Read the model definition and answer for the solid it produces. Units are mm, in the model's axes. A direction names the side the tool comes from. Coordinates: 2 decimals unless noted, no trailing zeros. Write each loop counter-clockwise with the first axis right and the second up, starting at its lowest first coordinate (ties: lowest second). Pieces come first, ordered by that corner, then holes.
Item 1: Each of these flat-tipped pins is pushed along its axis until it touches: P1, Ø1.9, axis at x = 0.5, y = -1, coming from the +Z side; P2, Ø1, axis at y = 1, z = -4, coming from the +X side. Where does it stop, or does it pass through?
Item 2: Section C-C (z = 2.25) is taken. Give the vertices of the cut face in (x, y), then the cut area to 3 significant figures.
Item 3: Section D-D (z = -10.75) is taken. Give the vertices of the cut face in (x, y).
Item 4: Determine the mould class of faces 1 (the face through (6.221, 0.028, 8.113)), 2 (the face through (-4.3, 2.032, 9.5)), 3 (the face through (0, 0, -12.7)), 4 (the face through (5, 0, 12.7)) for opening direction Z: released by +Z, released by -Z, zero draft, split by the parting line, or undercut.
Item 5: Straight lines are drawn through the part: probe 1 along X at (y, z) = (-0.2, 7.75); probe 2 along X at (y, z) = (0.4, 6.5); probe 3 along Z at (x, y) = (9, 1.3). For each, find the intervals that lie inside material, in ascending order.
Item 6: A tool of negligible diameter and unlimited length cuts with its end or side. For faces 5 (the face through (-11.05, 0.03, 6.26)), 6 (the face through (1.905, 0, 12)), from which of +Z, -Z, +X, -X, +Y, -Y can it reach the whole face along a straight path? Write none if from no direction.
Item 7: Section B-B (y = 0.55) is taken. Give the vertices of the cut face in (x, z) (1 decimal).
Item 8: Section A-A (x = 0) is taken. Give the vertices of the cut face in (y, z).
from build123d import *

# Parameters (mm, degrees)
SKETCH1_R           = 10.2235
BOSS_EXTRUDE1_DEPTH = 4.064


with BuildPart() as part:
    # Sketch1 → Boss-Extrude1 (new body)
    with BuildSketch(Plane(origin=(0, 2.032, 0), x_dir=(-1, 0, 0), z_dir=(0, 1, 0))):
        Polygon((1.905, 12.7), (1.905, 11.811), (-1.905, 11.811), (-1.905, 12.7), (-7.332348419, 12.7), (-14.664696837, 0), (-7.332348419, -12.7), (7.332348419, -12.7), (14.664696837, 0), (7.332348419, 12.7), align=None)
        with Locations(Location((0, 0, 0), (0, 0, 270))):
            Circle(SKETCH1_R, mode=Mode.SUBTRACT)
    extrude(amount=-BOSS_EXTRUDE1_DEPTH)


solid = part.part
Established:
1. P1: stops at z = 11.81
1. P2: stops at x = 12.64
2. outline: (-13.37, -2.03) - (-9.97, -2.03) - (-9.97, 2.03) - (-13.37, 2.03) - close; (9.97, -2.03) - (13.37, -2.03) - (13.37, 2.03) - (9.97, 2.03) - close
2. area: 27.6 mm2
3. outline: (-8.46, -2.03) - (8.46, -2.03) - (8.46, 2.03) - (-8.46, 2.03) - close
4. face 1: undercut
4. face 2: zero draft
4. face 3: released by -Z
4. face 4: released by +Z
5. probe 1: x = -10.19 to -6.67, 6.67 to 10.19
5. probe 2: x = -10.91 to -7.89, 7.89 to 10.91
5. probe 3: z = -9.81 to -4.85, 4.85 to 9.81
6. face 5: +Z, -X, +Y, -Y
6. face 6: +Z, +Y, -Y
7. outline: (-14.7, 0) - (-7.3, -12.7) - (7.3, -12.7) - (14.7, 0) - (7.3, 12.7) - (1.9, 12.7) - (1.9, 11.8) - (-1.9, 11.8) - (-1.9, 12.7) - (-7.3, 12.7) - close; hole circle Ø20.4 at (0, 0)
8. outline: (-2.03, -12.7) - (2.03, -12.7) - (2.03, -10.22) - (-2.03, -10.22) - close; (-2.03, 10.22) - (2.03, 10.22) - (2.03, 11.81) - (-2.03, 11.81) - close
